The model under review builds one solid part; all positions refer to its coordinate system, in mm. A direction names the side the tool comes from. Give positions to 0.01 mm unless a question says otherwise; leave off trailing zeros. Loops run counter-clockwise (first coordinate to the right, second up) from the corner with the lowest first, then second, coordinate; pieces in that order, holes last. Notation, with made-up numbers: (16, 75.5) - (66, 75.5) arc R26 ccw to (66, 92.5) - close; hole circle Ø1 at (50.25, -35). An arc over 180 degrees is marked (long way). Answer as a JSON object with one key per item and string values.
from build123d import *
from build123d.topology import SkipClean

# Parameters (mm, degrees)
SZKIC1_W                        = 48
SZKIC1_H                        = 142
DODANIE_WYCI_GNI_CIE1_DEPTH     = 4
DODANIE_WYCI_GNI_CIE3_DEPTH     = 4
WYTNIJ_WYCI_GNI_CIE1_DEPTH      = 55
WYTNIJ_WYCI_GNI_CIE1_DEPTH_BACK = 10
SZKIC3_R                        = 1.5
SZKIC4_W                        = 3
SZKIC4_H                        = 24.64
DODANIE_WYCI_GNI_CIE4_DEPTH     = 4
SZKIC5_W                        = 48
SZKIC5_H                        = 8
DODANIE_WYCI_GNI_CIE5_DEPTH     = 6
SZKIC6_W                        = 48
SZKIC6_H                        = 8
DODANIE_WYCI_GNI_CIE6_DEPTH     = 6
SZKIC9_R                        = 1.5
WYTNIJ_WYCI_GNI_CIE4_DEPTH      = 10
WYTNIJ_WYCI_GNI_CIE5_START      = -10
SZKIC10_R                       = 1.5
WYTNIJ_WYCI_GNI_CIE5_DEPTH      = 10
SZKIC12_W                       = 6.5
SZKIC12_H                       = 6.5
SZKIC12_R                       = 1.5
DODANIE_WYCI_GNI_CIE7_DEPTH     = 4
SZKIC15_R                       = 1.45
WYTNIJ_WYCI_GNI_CIE6_DEPTH      = 10
WYTNIJ_WYCI_GNI_CIE7_START      = -10
SZKIC16_R                       = 1.5
WYTNIJ_WYCI_GNI_CIE7_DEPTH      = 10
SFAZOWANIE1_SIZE                = 1


with BuildPart() as part:
    # Szkic1 → Dodanie-wyciągnięcie1 (new body)
    with BuildSketch(Plane.XY):
        with Locations((-11.283325816, 0)):
            Rectangle(SZKIC1_W, SZKIC1_H)
    extrude(amount=DODANIE_WYCI_GNI_CIE1_DEPTH)

    # Szkic2 → Dodanie-wyciągnięcie3 (add)
    with BuildSketch(Plane.XY.offset(4)):
        Polygon((-13.683325816, 12.317647524), (-19.283325816, 12.317647524), (-19.283325816, -12.322647524), (-16.483325816, -12.322647524), (-13.683325816, -12.322647524), align=None)
    extrude(amount=DODANIE_WYCI_GNI_CIE3_DEPTH)

    # Szkic3 → Wytnij-wyciągnięcie1 (cut, two sides: drawn at the far end of the back side and taken through both)
    with BuildSketch(Plane.XY.offset(8).offset(-WYTNIJ_WYCI_GNI_CIE1_DEPTH_BACK)):
        with Locations(Location((-16.483325816, 7.6225, 0), (0, 0, 180))):
            Circle(SZKIC3_R)
        with Locations(Location((-16.483325816, -7.6325, 0), (0, 0, 180))):
            Circle(SZKIC3_R)
    extrude(amount=WYTNIJ_WYCI_GNI_CIE1_DEPTH + WYTNIJ_WYCI_GNI_CIE1_DEPTH_BACK, mode=Mode.SUBTRACT)

    # Szkic4 → Dodanie-wyciągnięcie4 (add)
    with BuildSketch(Plane.XY.offset(4)):
        with Locations((-6.963325816, 0.250968311)):
            Rectangle(SZKIC4_W, SZKIC4_H)
    extrude(amount=DODANIE_WYCI_GNI_CIE4_DEPTH)

    # Szkic5 → Dodanie-wyciągnięcie5 (add)
    with BuildSketch(Plane.XY.offset(4)):
        with Locations((-11.283325816, 67)):
            Rectangle(SZKIC5_W, SZKIC5_H)
    extrude(amount=DODANIE_WYCI_GNI_CIE5_DEPTH)

    # Szkic6 → Dodanie-wyciągnięcie6 (add)
    with BuildSketch(Plane.XY.offset(4)):
        with Locations((-11.283325816, -67)):
            Rectangle(SZKIC6_W, SZKIC6_H)
    extrude(amount=DODANIE_WYCI_GNI_CIE6_DEPTH)

    # Szkic9 → Wytnij-wyciągnięcie4 (cut)
    with BuildSketch(Plane.XZ.offset(71)):
        with Locations(Location((-30.283325816, 7, 0), (0, 0, 270))):
            Circle(SZKIC9_R)
        with Locations(Location((7.716674184, 7, 0), (0, 0, 270))):
            Circle(SZKIC9_R)
    extrude(amount=-WYTNIJ_WYCI_GNI_CIE4_DEPTH, mode=Mode.SUBTRACT)

    # Szkic10 → Wytnij-wyciągnięcie5 (cut)
    with BuildSketch(Plane(origin=(0, 71, 0), x_dir=(-1, 0, 0), z_dir=(0, 1, 0)).offset(WYTNIJ_WYCI_GNI_CIE5_START)):
        with Locations(Location((-7.716674184, 7, 0), (0, 0, 270))):
            Circle(SZKIC10_R)
        with Locations(Location((30.283325816, 7, 0), (0, 0, 270))):
            Circle(SZKIC10_R)
    extrude(amount=WYTNIJ_WYCI_GNI_CIE5_DEPTH, mode=Mode.SUBTRACT)

    # Szkic12 → Dodanie-wyciągnięcie7 (add)
    # profile 1 of 2: a face of its own
    with BuildSketch(Plane.XY.offset(4)):
        with Locations((-19.283325816, 21.26353769)):
            Rectangle(SZKIC12_W, SZKIC12_H)
        with Locations((-19.283325816, 21.26353769)):
            Circle(SZKIC12_R, mode=Mode.SUBTRACT)
    # profile 2 of 2: a face of its own
    with BuildSketch(Plane.XY.offset(4)):
        with Locations((-3.283325816, 51.76353769)):
            Rectangle(SZKIC12_W, SZKIC12_H)
        with Locations((-3.283325816, 51.76353769)):
            Circle(SZKIC12_R, mode=Mode.SUBTRACT)
    extrude(amount=DODANIE_WYCI_GNI_CIE7_DEPTH)

    # Szkic15 → Wytnij-wyciągnięcie6 (cut)
    with BuildSketch(Plane.XY.offset(4)):
        with Locations((-11.283325816, -24.067309246)):
            Circle(SZKIC15_R)
        with Locations((-11.283325816, -43.567309246)):
            Circle(SZKIC15_R)
    extrude(amount=-WYTNIJ_WYCI_GNI_CIE6_DEPTH, mode=Mode.SUBTRACT)

    # Szkic16 → Wytnij-wyciągnięcie7 (cut)
    with SkipClean():  # the faces are left unmerged after this step: merging them gives an invalid solid
        with BuildSketch(Plane.XY.offset(8).offset(WYTNIJ_WYCI_GNI_CIE7_START)):
            with Locations(Location((-3.283325816, 51.76353769, 0), (0, 0, 180))):
                Circle(SZKIC16_R)
            with Locations(Location((-19.283325816, 21.26353769, 0), (0, 0, 180))):
                Circle(SZKIC16_R)
        extrude(amount=WYTNIJ_WYCI_GNI_CIE7_DEPTH, mode=Mode.SUBTRACT)

    # Sfazowanie1
    sfazowanie1_edges = [part.edges().sort_by_distance(p)[0] for p in [
        (-1.783325816, 51.76353769, 0),
        (-17.783325816, 21.26353769, 0),
        (-14.983325816, -7.6325, 0),
        (-14.983325816, 7.6225, 0),
    ]]
    chamfer(sfazowanie1_edges, length=SFAZOWANIE1_SIZE)


solid = part.part
Q1. For faces 5 (the face through (-7, -12.069, 6)), 6 (the face through (12.717, -1, 3)), 7 (the face through (-6.533, 52, 6)), 8 (the face through (-12, 63, 7)), 9 (the face through (-16.158, 9.087, 4.451)), list the 3-axis set-ups (+Z, -Z, +X, -X, +Y, -Y) from which the entire face can be reached by the end or side of a thin tool; tool diameter is ignored.
Results:
{"face 5": "+Z, +X", "face 6": "+Z, -Z, +X, +Y, -Y", "face 7": "+Z, -X", "face 8": "+Z, +X, -X", "face 9": "+Z, -Z"}
Q2. Consider section A-A, the plane x = 3.5. State the section outline as (y, z) points.
Results:
{"outline": "(-71, 0) - (71, 0) - (71, 10) - (63, 10) - (63, 4) - (-63, 4) - (-63, 10) - (-71, 10) - close"}
Q3. Clearance check with flat-ended pins moving along their axes: pin 1 Ø4.5 at (x, y) = (-17.5, -4) entering from +Z; pin 2 Ø1.2 at (y, z) = (-3, 6) entering from -X; pin 3 Ø3 at (y, z) = (22, 6) entering from -X. State where each tip first meets the part, or that it passes through.
Results:
{"pin 1": "stops at z = 8", "pin 2": "stops at x = -19.28", "pin 3": "stops at x = -22.53"}
Q4. Consider section B-B, the plane y = -38. State the section outline as (x, z) points.
Results:
{"outline": "(-35.28, 0) - (12.72, 0) - (12.72, 4) - (-35.28, 4) - close"}
Q5. The part is to be moulded in two halves that separate along X. For faces 1 (the face through (-17, -12.323, 6)), 2 (the face through (-12.73, -24, 2.03)), 3 (the face through (-13.683, 0, 6)), 4 (the face through (-0.033, 52, 6)), say which applies: +X half, -X half, draft (parallel to the pull), parting line (faces both ways), or undercut.
Results:
{"face 1": "draft", "face 2": "undercut", "face 3": "undercut", "face 4": "+X half"}
Q6. To check wall thickness, follow probe 1 along X at (y, z) = (-67.5, 7); probe 2 along Y at (x, z) = (-1, 4.75); probe 3 along Y at (x, z) = (4, 9.25). State the ranges of each line that lie inside material, in increasing order. Write a range as [from, to].
Results:
{"probe 1": "x = [-35.28, -31.78], [-28.78, 6.22], [9.22, 12.72]", "probe 2": "y = [-71, -63], [48.51, 55.01], [63, 71]", "probe 3": "y = [-71, -63], [63, 71]"}
